```python
from build123d import *

# Parameters (mm, degrees)
F1_DEPTH = 124
F3_START = -5
F2_W     = 114
F2_H     = 52
F3_DEPTH = 31.001
F4_SIZE  = 25


with BuildPart() as f1:
    # F0 (on Right) → F1 (new body)
    with BuildSketch(Plane.YZ):
        Polygon((-20, 36), (-20, 0), (37, 0), align=None)
    extrude(amount=F1_DEPTH)

    # F2 (on face) → F3 (cut)
    with BuildSketch(Plane(origin=(0, 0, 0), x_dir=(1, 0, 0), z_dir=(0, 0, -1)).offset(F3_START)):
        with Locations((62, -11)):
            Rectangle(F2_W, F2_H)
    extrude(amount=-F3_DEPTH, mode=Mode.SUBTRACT)

    # F4
    f4_edges = [f1.edges().sort_by_distance(p)[0] for p in [
        (62, -15, 5),
    ]]
    chamfer(f4_edges, length=F4_SIZE)


solid = f1.part
```
Design review of the part built by this model. Coordinates are the model's own, in mm. A direction names the side the tool comes from. Coordinates: 2 decimals unless noted, no trailing zeros. Write each loop counter-clockwise with the first axis right and the second up, starting at its lowest first coordinate (ties: lowest second). Pieces come first, ordered by that corner, then holes.
1) Insertion check: pin 1 (4 mm diameter, centred on x = 31, y = -9.5, fed in from +Z); pin 2 (8 mm diameter, centred on x = 84.5, y = -9, fed in from +Z); pin 3 (3 mm diameter, centred on x = 59, z = 31, fed in from +Y); pin 4 (14 mm diameter, centred on y = 1, z = 21, fed in from -X). Each pin has a flat end and moves straight along its axis. Give the tip position at first contact, or say it passes through.
2) To check wall thickness, follow L1, parallel to X at y = 16, z = 9; L2, parallel to Y at x = 113, z = 30; L3, parallel to Z at x = 83, y = 27.5. State the ranges of each line that lie inside material, in increasing order.
3) Add section C-C (z = 11.5). Write out the cut boundary in (x, y).
4) Add section A-A (x = 81). Write out the cut boundary in (y, z).
5) Machinability: for faces 5 (the flat face through (61, 8, 0)), 6 (the flat face through (61, -15, 31)), which of the approach directions +Z, -Z, +X, -X, +Y, -Y give a long, thin tool a straight path to every point of the face, cutting with its end or side? Answer none if there is none.
6) Add section D-D (z = 2.5). Write out the cut boundary in (x, y), plus the area to 3 significant figures.
7) Mouldability with a two-part tool opening along X and no side actions: class faces 1 (the flat face through (61, -3, 18)), 2 (the flat face through (124, -5, 10)), 3 (the flat face through (61, -20, 18)), 4 (the flat face through (119, 7, 15)) as +X half, -X half, draft (parallel to the pull), parting line (faces both ways), or undercut.
8) Add section B-B (y = 24). Write out the cut boundary in (x, z).
Check result:
1. pin 1: stops at z = 26.5
1. pin 2: stops at z = 28
1. pin 3: stops at y = -14.5
1. pin 4: stops at x = 0
2. L1: x = 0 to 5, 119 to 124
2. L2: y = -20 to -15
2. L3: z = 0 to 5
3. outline: (0, -20) - (124, -20) - (124, 18.79) - (119, 18.79) - (119, 3.5) - (5, 3.5) - (5, 18.79) - (0, 18.79) - close
4. outline: (-20, 0) - (37, 0) - (29.08, 5) - (10, 5) - (-15, 30) - (-15, 32.84) - (-20, 36) - close
5. face 5: -Z, +X, -X, +Y, -Y
5. face 6: +Z, +Y
6. outline: (0, -20) - (124, -20) - (124, 33.04) - (0, 33.04) - close
6. area: 6,580 mm2
7. face 1: undercut
7. face 2: +X half
7. face 3: draft
7. face 4: undercut
8. outline: (0, 0) - (124, 0) - (124, 8.21) - (119, 8.21) - (119, 5) - (5, 5) - (5, 8.21) - (0, 8.21) - close
